CAD build for the part. Positions are in the model's coordinates, mm. Face numbers are marked on the shaded views. Coordinates: 2 decimals unless noted, no trailing zeros. Order: outer loops, then holes, each group sorted by start corner. A loop starts at its lowest first (then second) coordinate and runs counter-clockwise, first axis right, second up. Notation, with made-up numbers: (40, 29) - (46, 29) arc R16 ccw to (46, 47) - close; hole circle Ø10 at (24.5, 19.5). An arc over 180 degrees is marked (long way). Return JSON: item names as keys, results as strings.
from build123d import *

# Parameters (mm, degrees)
SKETCH1_R               = 88.9
SKETCH1_R_2             = 82.55
BOSS_EXTRUDE1_DEPTH     = 25.4
SKETCH2_R               = 3.175
CUT_EXTRUDE1_DEPTH      = 89.9
CUT_EXTRUDE1_DEPTH_BACK = 89.9
SKETCH3_R               = 2.159
CUT_EXTRUDE2_DEPTH      = 89.9000001
CUT_EXTRUDE2_DEPTH_BACK = 89.9000001


with BuildPart() as part:
    # Sketch1 → Boss-Extrude1 (new body)
    with BuildSketch(Plane(origin=(0, 0, 0), x_dir=(1, 0, 0), z_dir=(0, 1, 0))):
        Circle(SKETCH1_R)
        Circle(SKETCH1_R_2, mode=Mode.SUBTRACT)
    extrude(amount=BOSS_EXTRUDE1_DEPTH)

    # Sketch2 → Cut-Extrude1 (cut, two sides)
    with BuildSketch(Plane(origin=(0, 0, 0), x_dir=(0, 0, -1), z_dir=(1, 0, 0))) as cut_extrude1_sk:
        with Locations((0, 12.7)):
            Circle(SKETCH2_R)
    extrude(amount=CUT_EXTRUDE1_DEPTH, mode=Mode.SUBTRACT)
    extrude(cut_extrude1_sk.sketch, amount=-CUT_EXTRUDE1_DEPTH_BACK, mode=Mode.SUBTRACT)

    # Sketch3 → Cut-Extrude2 (cut, two sides)
    with BuildSketch(Plane.XY) as cut_extrude2_sk:
        with Locations((0, 12.7)):
            Circle(SKETCH3_R)
    extrude(amount=CUT_EXTRUDE2_DEPTH, mode=Mode.SUBTRACT)
    extrude(cut_extrude2_sk.sketch, amount=-CUT_EXTRUDE2_DEPTH_BACK, mode=Mode.SUBTRACT)


solid = part.part
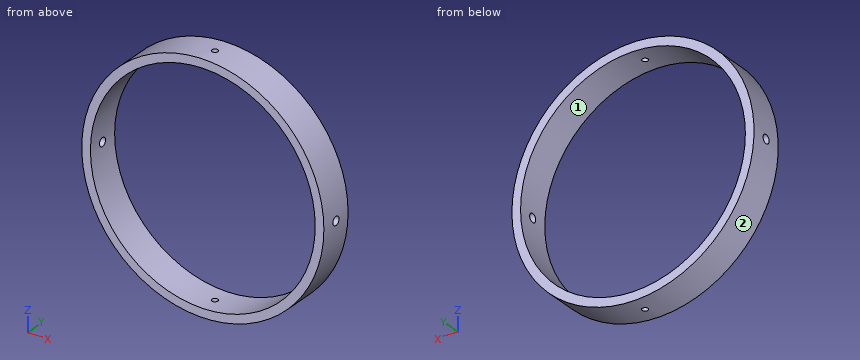
Item 1: Wall check: L1, parallel to Z at x = 0, y = 10.5; L2, parallel to Y at x = -86, z = 0 (3 decimals); L3, parallel to X at y = 14, z = 3. Give the ranges that are in metal, low to high. Write a range as [from, to].
Findings below:
{"L1": "z = [-88.9, -82.55], [82.55, 88.9]", "L2": "y = [0, 9.525], [15.875, 25.4]", "L3": "x = [-88.85, -82.5], [82.5, 88.85]"}
Item 2: Band-saw the part on D-D, the plane x = 74.5. List the corners of the cut face in (y, z).
Findings below:
{"outline": "(0, -48.51) - (25.4, -48.51) - (25.4, -35.56) - (0, -35.56) - close; (0, 35.56) - (25.4, 35.56) - (25.4, 48.51) - (0, 48.51) - close"}
Item 3: Band-saw the part on C-C, the plane z = 39. List the corners of the cut face in (x, y), then the cut area to 3 significant figures.
Findings below:
{"outline": "(-79.89, 0) - (-72.76, 0) - (-72.76, 25.4) - (-79.89, 25.4) - close; (72.76, 0) - (79.89, 0) - (79.89, 25.4) - (72.76, 25.4) - close", "area": "362 mm²"}
Item 4: Band-saw the part on A-A, the plane x = 0. List the corners of the cut face in (y, z), then the cut area to 3 significant figures.
Findings below:
{"outline": "(0, -88.9) - (10.54, -88.9) - (10.54, -82.55) - (0, -82.55) - close; (0, 82.55) - (10.54, 82.55) - (10.54, 88.9) - (0, 88.9) - close; (14.86, -88.9) - (25.4, -88.9) - (25.4, -82.55) - (14.86, -82.55) - close; (14.86, 82.55) - (25.4, 82.55) - (25.4, 88.9) - (14.86, 88.9) - close", "area": "268 mm²"}
Item 5: Band-saw the part on B-B, the plane z = 0. List the corners of the cut face in (x, y) (3 decimals).
Findings below:
{"outline": "(-88.9, 0) - (-82.55, 0) - (-82.55, 9.525) - (-88.9, 9.525) - close; (-88.9, 15.875) - (-82.55, 15.875) - (-82.55, 25.4) - (-88.9, 25.4) - close; (82.55, 0) - (88.9, 0) - (88.9, 9.525) - (82.55, 9.525) - close; (82.55, 15.875) - (88.9, 15.875) - (88.9, 25.4) - (82.55, 25.4) - close"}
Item 6: Mould opens along X. For the marked faces 1 and 2 say: released by +X, released by -X, zero draft, split by the parting line, or undercut.
Findings below:
{"face 1": "undercut", "face 2": "split by the parting line"}
Item 7: Drop flat-ended pins along their axis: P1, Ø5, axis at y = 18, z = -58.5, coming from the +X side (3 decimals); P2, Ø3, axis at y = 4.5, z = -25.5, coming from the -X side; P3, Ø1, axis at y = 12, z = -43.5, coming from the -X side. Give the stop position or say it passes through.
Findings below:
{"P1": "stops at x = 69.045", "P2": "stops at x = -85.6", "P3": "stops at x = -77.81"}
